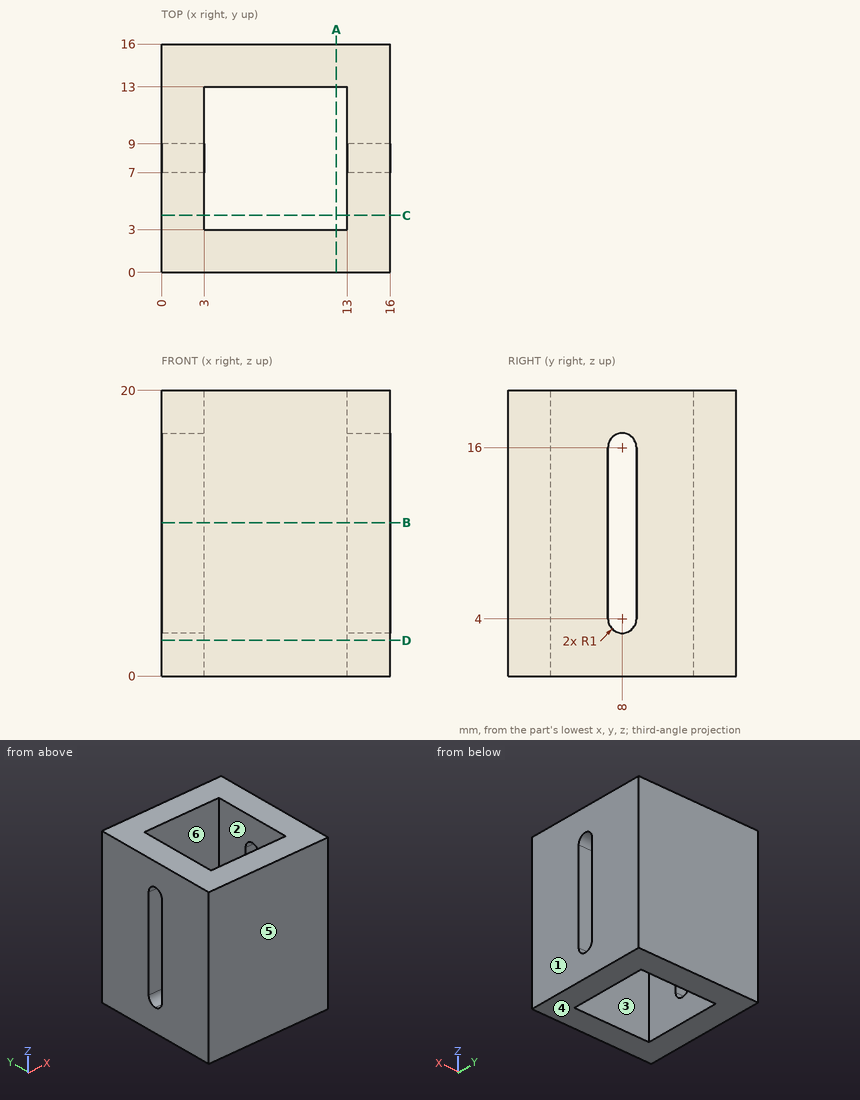
For this review, use the dimensioned drawing (mm, ordinates from the lowest corner) and the shaded views. A direction names the side the tool comes from. Coordinates: 2 decimals unless noted, no trailing zeros. Write each loop counter-clockwise with the first axis right and the second up, starting at its lowest first coordinate (ties: lowest second). Pieces come first, ordered by that corner, then holes. Notation, with made-up numbers: (31, 28.25) - (41, 28.25) arc R5 ccw to (41, 33.25) - close; hole circle Ø10 at (33, 7). An arc over 180 degrees is marked (long way). One line per item, written item: value.
1) To check wall thickness, follow probe 1 along Y at (x, z) = (10, 6); probe 2 along Y at (x, z) = (1, 13). State the ranges of each line that lie inside material, in increasing order.
Answer sheet:
probe 1: y = 0 to 3, 13 to 16
probe 2: y = 0 to 7, 9 to 16
2) Insertion check: pin 1 (2 mm diameter, centred on x = 9.5, y = 11, fed in from +Z). The pin has a flat end and moves straight along its axis. Give the tip position at first contact, or say it passes through.
Answer sheet:
pin 1: passes through
3) Add section A-A (x = 12.25). State the section outline as (y, z) points, plus the area to 3 significant figures.
Answer sheet:
outline: (0, 0) - (3, 0) - (3, 20) - (0, 20) - close; (13, 0) - (16, 0) - (16, 20) - (13, 20) - close
area: 120 mm2
4) Mouldability with a two-part tool opening along X and no side actions: class the marked faces 1, 2, 3 and 4 as +X half, -X half, draft (parallel to the pull), parting line (faces both ways), or undercut.
Answer sheet:
face 1: +X half
face 2: undercut
face 3: undercut
face 4: draft
5) Add section D-D (z = 2.5). State the section outline as (x, y) points.
Answer sheet:
outline: (0, 0) - (16, 0) - (16, 16) - (0, 16) - close; hole (3, 3) - (13, 3) - (13, 13) - (3, 13) - close
6) For the marked faces 5 and 6, list the 3-axis set-ups (+Z, -Z, +X, -X, +Y, -Y) from which the entire face can be reached by the end or side of a thin tool; tool diameter is ignored.
Answer sheet:
face 5: +Z, -Z, +X, -X, -Y
face 6: +Z, -Z
7) Add section B-B (z = 10.75). State the section outline as (x, y) points, plus the area to 3 significant figures.
Answer sheet:
outline: (0, 0) - (16, 0) - (16, 7) - (13, 7) - (13, 3) - (3, 3) - (3, 7) - (0, 7) - close; (0, 9) - (3, 9) - (3, 13) - (13, 13) - (13, 9) - (16, 9) - (16, 16) - (0, 16) - close
area: 144 mm2
